Geometry check sheet. Reference: drawing and pictorial views, mm from the part's lowest x, y, z. Give positions to 0.01 mm unless a question says otherwise; leave off trailing zeros. Order: outer loops, then holes, each group sorted by start corner. A loop starts at its lowest first (then second) coordinate and runs counter-clockwise, first axis right, second up.
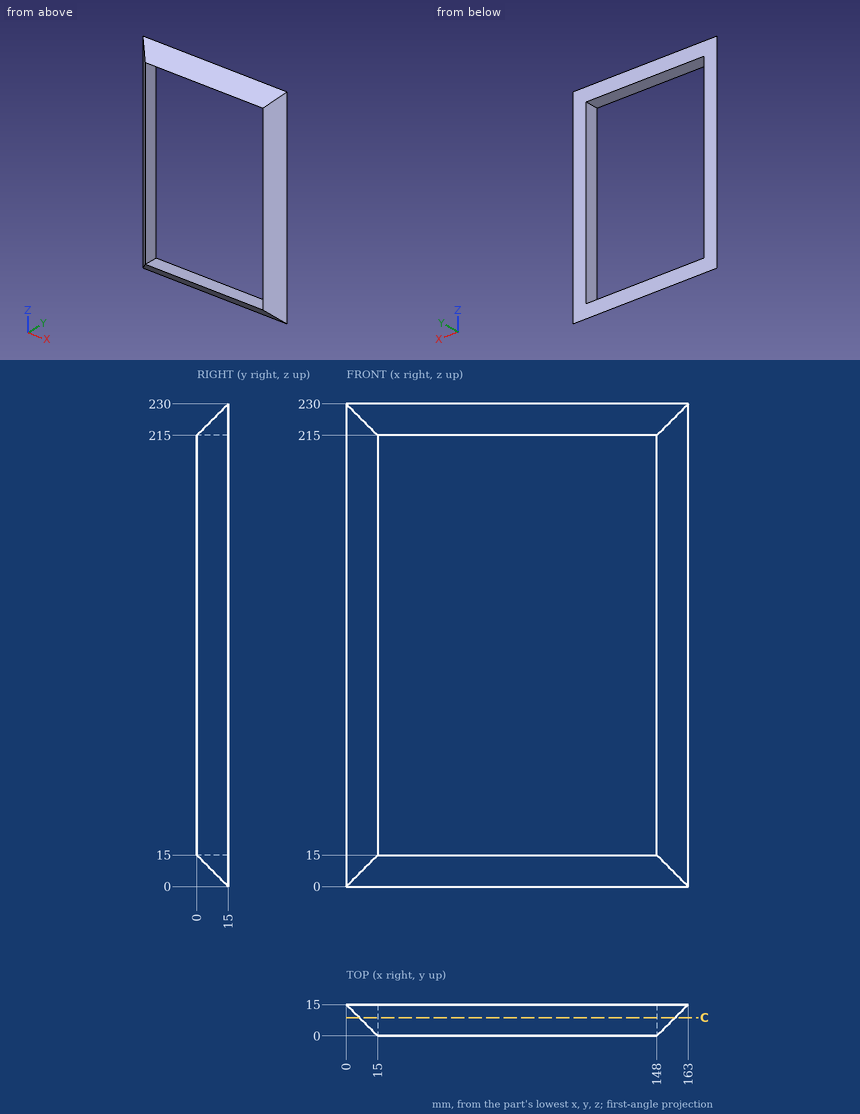
(1) Go/stop test with flat-tipped pins: P1, Ø1.5, axis at x = 27.5, y = 2, coming from the +Z side; P2, Ø6, axis at y = 9, z = 195.5, coming from the +X side; P3, Ø6, axis at x = 43.5, y = 9.5, coming from the +Z side. Record where each tip stops, or that it passes through.
(2) Sectioned sample at C-C (y = 8.75). Enter the section's corners in (x, z), plus the area to 3 significant figures.
(3) Thickness scan on L1, parallel to X at y = 14.25, z = 105; L2, parallel to Z at x = 88, y = 1.5; L3, parallel to Z at x = 101, y = 2.25. Record the ranges inside material, lowest first.
Values follow:
1. P1: stops at z = 217.75
1. P2: stops at x = 160
1. P3: stops at z = 227.5
2. outline: (6.25, 6.25) - (156.75, 6.25) - (156.75, 223.75) - (6.25, 223.75) - close; hole (15, 15) - (148, 15) - (148, 215) - (15, 215) - close
2. area: 6,130 mm2
3. L1: x = 0.75 to 15, 148 to 162.25
3. L2: z = 13.5 to 15, 215 to 216.5
3. L3: z = 12.75 to 15, 215 to 217.25
